Part print with two shaded views. Sizes in mm from the minimum x, y, z corner. A direction names the side the tool comes from. Coordinates: 2 decimals unless noted, no trailing zeros. Write each loop counter-clockwise with the first axis right and the second up, starting at its lowest first coordinate (ties: lowest second). Pieces come first, ordered by that corner, then holes. Notation, with made-up numbers: (24.25, -5.5) - (44.25, -5.5) arc R35 cw to (44.25, 31.5) - close; hole circle Ø5 at (72.5, 39). An arc over 180 degrees is marked (long way). One line per question, with ' | ' between items. Start each with the question number.
1. Flat gauge pins, fed straight in: P1, Ø1, axis at y = 38, z = 20.5, coming from the +X side; P2, Ø12, axis at x = 15.5, z = 20.5, coming from the +Y side; P3, Ø20, axis at x = 62.5, z = 22.5, coming from the -Y side. Where does each tip first touch, or does it go through?
2. Band-saw the part on C-C, the plane x = 35. Write the cut outline in (y, z), then the cut area to 3 significant figures.
3. Band-saw the part on A-A, the plane z = 16. Write the cut outline in (x, y) (1 decimal).
4. Band-saw the part on B-B, the plane y = 36. Write the cut outline in (x, z), then the cut area to 3 significant figures.
5. Two-plate mould, pull along Y, no slides. Class the marked faces 1, 2 and 3: +Y half, -Y half, draft (parallel to the pull), parting line (faces both ways), or undercut.
6. Band-saw the part on D-D, the plane y = 24. Write the cut outline in (x, z) (1 decimal), then the cut area to 3 significant figures.
7. Probe line 1 (Y direction, x = 72, z = 21); line 2 (X direction, y = 26, z = 27.5) (1 decimal); line 3 (Z direction, x = 29, y = 31). List the from-to ranges inside material, lowest first.
8. Which spindle directions (+Z, -Z, +X, -X, +Y, -Y) get a long thin tool onto all of the face, cutting with end or side? Do the marked faces 4, 5, 6, 7 and 8. Say none if no direction does.
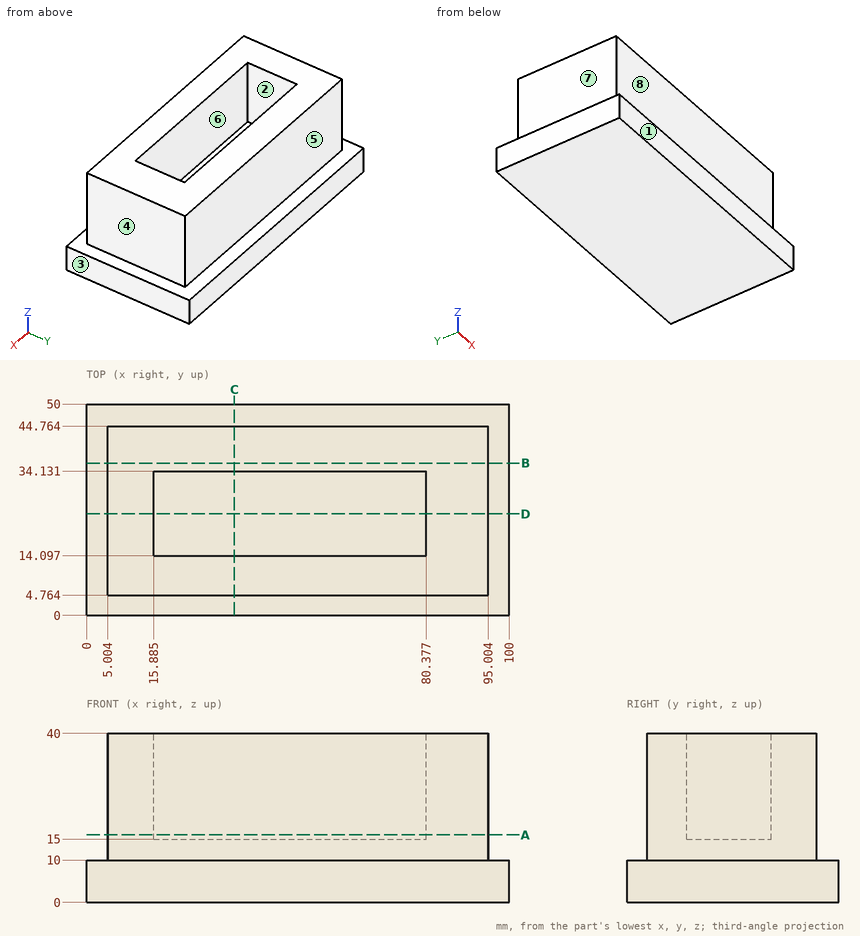
Filled in:
1) P1: stops at x = 95 | P2: stops at y = 44.76 | P3: stops at y = 4.76
2) outline: (0, 0) - (50, 0) - (50, 10) - (44.76, 10) - (44.76, 40) - (34.13, 40) - (34.13, 15) - (14.1, 15) - (14.1, 40) - (4.76, 40) - (4.76, 10) - (0, 10) - close | area: 1,200 mm²
3) outline: (5, 4.8) - (95, 4.8) - (95, 44.8) - (5, 44.8) - close; hole (15.9, 14.1) - (80.4, 14.1) - (80.4, 34.1) - (15.9, 34.1) - close
4) outline: (0, 0) - (100, 0) - (100, 10) - (95, 10) - (95, 40) - (5, 40) - (5, 10) - (0, 10) - close | area: 3,700 mm²
5) face 1: -Y half | face 2: undercut | face 3: draft
6) outline: (0, 0) - (100, 0) - (100, 10) - (95, 10) - (95, 40) - (80.4, 40) - (80.4, 15) - (15.9, 15) - (15.9, 40) - (5, 40) - (5, 10) - (0, 10) - close | area: 2,090 mm²
7) line 1: y = 4.76 to 14.1, 34.13 to 44.76 | line 2: x = 5 to 15.9, 80.4 to 95 | line 3: z = 0 to 15
8) face 4: +Z, +X, +Y, -Y | face 5: +Z, +X, -X, +Y | face 6: +Z | face 7: +Z, -X, +Y, -Y | face 8: +Z, +X, -X, -Y
